Can you work these out from the model? Positions are in its coordinate system, mm. A direction names the side the tool comes from. Give positions to 0.01 mm unless a question says otherwise; leave off trailing zeros. Write each loop counter-clockwise with the first axis right and the second up, starting at its lowest first coordinate (ties: lowest second). Pieces come first, ordered by that corner, then holes.
1. Suppose I cut it at B-B (y = 21.5). Please give me the cut outline in (x, z).
2. I'm going to push flat-ended pins straight in: pin 1 (12 mm diameter, centred on x = 65.5, y = 23, fed in from -Z); pin 2 (1.1 mm diameter, centred on y = -0.5, z = 24, fed in from +X); pin 3 (2 mm diameter, centred on y = 28, z = -8, fed in from -X); pin 4 (10 mm diameter, centred on y = 12.5, z = 1.5, fed in from +X). Where does each tip first touch, or does it pass through?
3. On a 3-axis mill with a long thin cutter (end or side, diameter ignored), from which of +Z, -Z, +X, -X, +Y, -Y can I reach the whole of each face in a straight line? I mean faces 4 (the cylindrical face through (19.806, 0.07, -23.212)), 5 (the flat face through (102, 8, 8.001)), 6 (the flat face through (102, 8, -8.001)). Say none if no direction works.
4. If I drill on probe 1 along Z at (x, y) = (50, 2); probe 2 along Y at (x, z) = (55, -11); probe 3 along X at (y, z) = (-2, 25.4), over which ranges is the centre line in solid material (lowest first)?
5. Suppose I cut it at A-A (z = 0). Give the number of separate pieces and of enclosed holes in the cut face, and give its area (3 significant figures).
6. Thinking about a two-plate mould opening in X: for faces 1 (the cylindrical face through (73.18, 0.07, -12.584)), 2 (the cylindrical face through (44.95, -0.07, 24.1)), 3 (the cylindrical face through (57.12, 0.07, 42.29)), which applies, pulls with the +X half, pulls with the -X half, needs draft (parallel to the pull), parting line crosses it, or undercut?
7. Suppose I cut it at D-D (x = 4). Please give me the cut outline in (y, z), and give its area (3 significant figures).
8. Suppose I cut it at C-C (y = 2). Please give me the cut outline in (x, z), and give its area (3 significant figures).
```python
from build123d import *

# Parameters (mm, degrees)
SKETCH2_R           = 5.9944
BOSS_EXTRUDE1_DEPTH = 5.0038
SKETCH3_R           = 9.9695
BOSS_EXTRUDE2_DEPTH = 8.001
FILLET1_R           = 15.24


with BuildPart() as part:
    # Sketch2 → Boss-Extrude1 (new, symmetric)
    with BuildSketch(Plane(origin=(0, 0, 0), x_dir=(1, 0, 0), z_dir=(0, 1, 0))):
        with BuildLine():
            Line((68.834, 25.4), (68.834, -25.4))
            ThreePointArc((68.834, -25.4), (56.830149579, -42.395953991), (36.798683148, -36.76610234))
            ThreePointArc((36.798683148, -36.76610234), (20.076804637, -23.346390726), (-0.69209176, -18.020714886))
            ThreePointArc((-0.69209176, -18.020714886), (-18.034, 0), (-0.69209176, 18.020714886))
            ThreePointArc((-0.69209176, 18.020714886), (20.076804637, 23.346390726), (36.798683148, 36.76610234))
            ThreePointArc((36.798683148, 36.76610234), (56.830149579, 42.395953991), (68.834, 25.4))
        make_face()
        with Locations(Location((0, 0, 0), (0, 0, 270))):
            Circle(SKETCH2_R, mode=Mode.SUBTRACT)
        with Locations(Location((50.8, 25.4, 0), (0, 0, 270))):
            Circle(SKETCH2_R, mode=Mode.SUBTRACT)
        with Locations(Location((50.8, -25.4, 0), (0, 0, 270))):
            Circle(SKETCH2_R, mode=Mode.SUBTRACT)
    extrude(amount=BOSS_EXTRUDE1_DEPTH, both=True)

    # Sketch3 → Boss-Extrude2 (add, symmetric)
    with BuildSketch(Plane.XY):
        with BuildLine():
            Line((109.855, -5.0038), (68.834, -5.0038))
            Line((68.834, -5.0038), (68.834, 5.0038))
            Line((68.834, 5.0038), (36.798683148, 5.0038))
            Line((36.798683148, 5.0038), (19.200610133, 5.0038))
            ThreePointArc((19.200610133, 5.0038), (59.795544448, 12.455583787), (95.097308626, 33.839297674))
            ThreePointArc((95.097308626, 33.839297674), (130.631042041, 25.11465945), (109.855, -5.0038))
        make_face()
        with Locations((109.855, 17.2212)):
            Circle(SKETCH3_R, mode=Mode.SUBTRACT)
    extrude(amount=BOSS_EXTRUDE2_DEPTH, both=True)

    # Fillet1
    fillet1_edges = [part.edges().sort_by_distance(p)[0] for p in [
        (68.834, 0, 8.001),
        (68.834, 0, -8.001),
    ]]
    fillet(fillet1_edges, radius=FILLET1_R)


solid = part.part
```
Checks:
1. outline: (78.35, -8) - (100.85, -8) - (100.85, 8) - (78.35, 8) - close; (118.86, -8) - (131.66, -8) - (131.66, 8) - (118.86, 8) - close
2. pin 1: passes through
2. pin 2: stops at x = 68.83
2. pin 3: stops at x = 86.61
2. pin 4: stops at x = 132.08
3. face 4: -Z, -X, +Y, -Y
3. face 5: +Z, +X, +Y
3. face 6: -Z, +X, +Y
4. probe 1: z = -43.42 to -31.34, -19.46 to 19.46, 31.34 to 43.42
4. probe 2: y = -5 to 5
4. probe 3: x = 23.79 to 44.81, 56.79 to 68.83
5. separate pieces: 2
5. enclosed holes: 1
5. area: 2,790 mm2
6. face 1: pulls with the +X half
6. face 2: undercut
6. face 3: parting line crosses it
7. outline: (-5, -18.42) - (5, -18.42) - (5, -4.46) - (-5, -4.46) - close; (-5, 4.46) - (5, 4.46) - (5, 18.42) - (-5, 18.42) - close
7. area: 279 mm2
8. outline: (-0.69, -18.02) arc R50.8 cw to (36.8, -36.77) arc R18.03 ccw to (68.83, -25.4) - (68.83, -23.24) arc R15.24 cw to (84.07, -8) - (126.05, -8) - (126.05, 8) - (84.07, 8) arc R15.24 cw to (68.83, 23.24) - (68.83, 25.4) arc R18.03 ccw to (36.8, 36.77) arc R50.8 cw to (-0.69, 18.02) arc R18.03 ccw to start; hole circle Ø11.99 at (0, 0); hole circle Ø11.99 at (50.8, -25.4); hole circle Ø11.99 at (50.8, 25.4)
8. area: 5,550 mm2
